Design review of the part built by this model. Coordinates are the model's own, in mm. A direction names the side the tool comes from. Coordinates: 2 decimals unless noted, no trailing zeros. Loops run counter-clockwise (first coordinate to the right, second up) from the corner with the lowest first, then second, coordinate; pieces in that order, holes last. Notation, with made-up numbers: (-11.75, -21) -> (40.25, -21) arc R20 ccw to (40.25, 0) -> close; hole circle Ø7 at (84, -1). An arc over 180 degrees is marked (long way). One line per item, written item: value. Start each with the question number.
1. Draft analysis for pull direction Y (two halves, no side actions). For faces 4 (the flat face through (46.052, -18, 15)), 5 (the cylindrical face through (41.581, -11.097, -0.563)), 6 (the flat face through (3, -13.616, -13)), state which applies: pulls with the +Y half, pulls with the -Y half, needs draft (parallel to the pull), parting line crosses it, or undercut.
2. Add section D-D on y = -22.75. Write out the cut boundary in (x, z).
3. Add section B-B on y = -3.5. Write out the cut boundary in (x, z), plus the area to 3 significant figures.
4. Machinability: for faces 1 (the cylindrical face through (-34.55, -11.097, -0.563)), 2 (the flat face through (3, -13.616, 31)), 3 (the flat face through (4, -15, -9.76)), which of the approach directions +Z, -Z, +X, -X, +Y, -Y give a long, thin tool a straight path to every point of the face, cutting with its end or side? Answer none if there is none.
5. For probe 1 along Z at (x, y) = (-21, -23.25); probe 2 along X at (y, z) = (-19, 14); probe 3 along X at (y, z) = (-7.75, -10.5), list the stretches that pass through material, from the lowest coordinate up.
6. Add section C-C on z = 17.5. Write out the cut boundary in (x, y), plus the area to 3 significant figures.
7. Insertion check: pin 1 (10 mm diameter, centred on y = -12.88, z = 7.48, fed in from -X); pin 2 (2.5 mm diameter, centred on x = 8, z = 30, fed in from +Y). Each pin has a flat end and moves straight along its axis. Give the tip position at first contact, or say it passes through.
8. Add section A-A on x = 20. Write out the cut boundary in (y, z).
```python
from build123d import *

# Parameters (mm, degrees)
F0_W     = 66.0323537886
F0_H     = 6.7478315905
F1_DEPTH = 25.4
F2_DEPTH = 25.4
F3_W     = 26.5093389899
F3_H     = 13.6161595583
F4_DEPTH = 76.454
F5_R     = 8.2379774364
F6_DEPTH = 155.194


with BuildPart() as f1:
    # F0 (on Front) → F1 (new body)
    with BuildSketch(Plane.XZ):
        Polygon((-40.1414297521, 27.1496288478), (-28.7987813354, 27.1496288478), (37.2335724533, 27.1496288478), (37.2335724533, 35.2556668222), (-40.1414297521, 35.2556668222), align=None)
        with Locations((4.217395559, -13.1341717206)):
            Rectangle(F0_W, F0_H)
        Polygon((-40.1414297521, -16.5080875158), (-28.7987813354, -16.5080875158), (-28.7987813354, -9.7602559254), (-28.7987813354, 27.1496288478), (-40.1414297521, 27.1496288478), align=None)
        Polygon((37.2335724533, -9.7602559254), (37.2335724533, -16.5080875158), (46.05165869, -16.5080875158), (46.05165869, 35.2556668222), (37.2335724533, 35.2556668222), (37.2335724533, 27.1496288478), align=None)
    extrude(amount=F1_DEPTH)

    # F0 (on Front) → F2 (join)
    with BuildSketch(Plane.XZ):
        Polygon((-40.1414297521, 27.1496288478), (-28.7987813354, 27.1496288478), (37.2335724533, 27.1496288478), (37.2335724533, 35.2556668222), (-40.1414297521, 35.2556668222), align=None)
        with Locations((4.217395559, -13.1341717206)):
            Rectangle(F0_W, F0_H)
        Polygon((-40.1414297521, -16.5080875158), (-28.7987813354, -16.5080875158), (-28.7987813354, -9.7602559254), (-28.7987813354, 27.1496288478), (-40.1414297521, 27.1496288478), align=None)
        Polygon((37.2335724533, -9.7602559254), (37.2335724533, -16.5080875158), (46.05165869, -16.5080875158), (46.05165869, 35.2556668222), (37.2335724533, 35.2556668222), (37.2335724533, 27.1496288478), align=None)
    extrude(amount=F2_DEPTH)

    # F3 (on face) → F4 (cut)
    with BuildSketch(Plane.XY.offset(35.2556668222)):
        with Locations((2.7714306489, -6.8080797791)):
            Rectangle(F3_W, F3_H)
    extrude(amount=-F4_DEPTH, mode=Mode.SUBTRACT)

    # F5 (on face) → F6 (cut)
    with BuildSketch(Plane(origin=(-40.1414297521, 0, 0), x_dir=(0, -1, 0), z_dir=(-1, 0, 0))):
        with Locations((12.8824114799, 7.4787386693)):
            Circle(F5_R)
    extrude(amount=-F6_DEPTH, mode=Mode.SUBTRACT)


solid = f1.part
```
Worked answers:
1. face 4: needs draft
1. face 5: undercut
1. face 6: pulls with the +Y half
2. outline: (-40.14, -16.51) -> (46.05, -16.51) -> (46.05, 35.26) -> (-40.14, 35.26) -> close; hole (-28.8, -9.76) -> (37.23, -9.76) -> (37.23, 27.15) -> (-28.8, 27.15) -> close
3. outline: (-40.14, -16.51) -> (-10.48, -16.51) -> (-10.48, -9.76) -> (-28.8, -9.76) -> (-28.8, 27.15) -> (-10.48, 27.15) -> (-10.48, 35.26) -> (-40.14, 35.26) -> close; (16.03, -16.51) -> (46.05, -16.51) -> (46.05, 35.26) -> (16.03, 35.26) -> (16.03, 27.15) -> (37.23, 27.15) -> (37.23, -9.76) -> (16.03, -9.76) -> close
3. area: 1,630 mm²
4. face 1: +X, -X
4. face 2: +Z, -Z, +Y
4. face 3: +Y, -Y
5. probe 1: z = -16.51 to -9.76, 27.15 to 35.26
5. probe 2: x = -40.14 to -28.8, 37.23 to 46.05
5. probe 3: x = -40.14 to -10.48, 16.03 to 46.05
6. outline: (-40.14, -25.4) -> (-28.8, -25.4) -> (-28.8, 0) -> (-40.14, 0) -> close; (37.23, -25.4) -> (46.05, -25.4) -> (46.05, 0) -> (37.23, 0) -> close
6. area: 512 mm²
7. pin 1: passes through
7. pin 2: stops at y = -13.62
8. outline: (-25.4, -16.51) -> (0, -16.51) -> (0, -9.76) -> (-25.4, -9.76) -> close; (-25.4, 27.15) -> (0, 27.15) -> (0, 35.26) -> (-25.4, 35.26) -> close
